Here's how the part is built. I have some questions about the finished solid (model axes, mm). A direction names the side the tool comes from. Round coordinates to 2 decimals unless told otherwise and drop trailing zeros. Write each loop counter-clockwise with the first axis right and the second up, starting at its lowest first coordinate (ties: lowest second). Pieces come first, ordered by that corner, then holes. Notation, with made-up numbers: M 56,36.5 L 96,36.5 A37 cw 96,73.5 Z; hole C 66.5,83.25 d11. An arc over 180 degrees is marked long. Write item = value, one per line. Start each with the question number.
(1) I want a section at C-C (z = -2). Give the number of separate pieces and of enclosed holes in the cut face, and give its area (3 significant figures).
(2) If we mould it in two halves opening along Y, with no side actions, what happens to faces 4 (the flat face through (0, 7, 2)), 5 (the flat face through (-13, 1.55, 1)), 6 (the flat face through (-12.1, 5, -2)), 7 (the flat face through (0, 10, -2))? For each: released by +Y, released by -Y, zero draft, split by the parting line, or undercut.
(3) I want a section at A-A (x = 7). List the corners of the cut face in (y, z) for me.
(4) I want a section at D-D (x = 16). List the corners of the cut face in (y, z) for me, and give its area (3 significant figures).
(5) I want a section at B-B (y = -4.75). List the corners of the cut face in (x, z) for me, and give its area (3 significant figures).
(6) I need wall thicknesses on line 1 along X through (y, z) = (7.55, -2); line 2 along X through (y, z) = (-8.55, -2); line 3 along X through (y, z) = (5, -4.25). Which ranges of each line are inside material? Lowest first, please.
(7) Will this pin go through, and if not, where does the flat tip stop? pin 1 Ø4.5 at (x, y) = (-14.5, 1) entering from -Z.
(8) On a 3-axis mill with a long thin cutter (end or side, diameter ignored), from which of +Z, -Z, +X, -X, +Y, -Y can I reach the whole of each face in a straight line? I mean faces 1 (the flat face through (0, -6.2, 1)), 2 (the flat face through (0, 8.02, -3)), 3 (the flat face through (0, -10, -2)). Say none if no direction works.
```python
from build123d import *

# Parameters (mm, degrees)
SKETCH_1_W          = 40
SKETCH_1_H          = 20
EXTRUDE_1_DEPTH     = 2
SKETCH_2_W          = 24.2
SKETCH_2_H          = 12.4
CUT_EXTRUDE_1_DEPTH = 2
SKETCH_3_W          = 2
SKETCH_3_H          = 20
EXTRUDE_2_DEPTH     = 6
SKETCH_5_W          = 36
SKETCH_5_H          = 1.98
EXTRUDE_3_DEPTH     = 6
SKETCH_6_W          = 5.9
SKETCH_6_H          = 4
EXTRUDE_4_DEPTH     = 6
SKETCH_7_R          = 1.2
CUT_EXTRUDE_2_DEPTH = 29.91366459


with BuildPart() as part:
    # ｽｹｯﾁ1 → ﾎﾞｽ - 押し出し1 (new body)
    with BuildSketch(Plane.XY):
        Rectangle(SKETCH_1_W, SKETCH_1_H)
    extrude(amount=EXTRUDE_1_DEPTH)

    # ｽｹｯﾁ2 → ｶｯﾄ - 押し出し1 (cut)
    with BuildSketch(Plane.XY.offset(2)):
        Rectangle(SKETCH_2_W, SKETCH_2_H)
        with BuildLine():
            Line((-14, 1.55), (14, 1.55))
            ThreePointArc((14, 1.55), (15.55, 0), (14, -1.55))
            Line((14, -1.55), (-14, -1.55))
            ThreePointArc((-14, -1.55), (-15.55, 0), (-14, 1.55))
        make_face()
    extrude(amount=-CUT_EXTRUDE_1_DEPTH, mode=Mode.SUBTRACT)

    # ｽｹｯﾁ3 → ﾎﾞｽ - 押し出し2 (add)
    with BuildSketch(Plane(origin=(0, 0, 0), x_dir=(-1, 0, 0), z_dir=(0, 0, -1))):
        with Locations((19, 0)):
            Rectangle(SKETCH_3_W, SKETCH_3_H)
        with Locations((-19, 0)):
            Rectangle(SKETCH_3_W, SKETCH_3_H)
    extrude(amount=EXTRUDE_2_DEPTH)

    # ｽｹｯﾁ5 → ﾎﾞｽ - 押し出し3 (add)
    with BuildSketch(Plane(origin=(0, 0, 0), x_dir=(-1, 0, 0), z_dir=(0, 0, -1))):
        with Locations((0, 9.01)):
            Rectangle(SKETCH_5_W, SKETCH_5_H)
        with Locations((0, -9.01)):
            Rectangle(SKETCH_5_W, SKETCH_5_H)
    extrude(amount=EXTRUDE_3_DEPTH)

    # ｽｹｯﾁ6 → ﾎﾞｽ - 押し出し4 (add)
    with BuildSketch(Plane(origin=(0, 0, 0), x_dir=(-1, 0, 0), z_dir=(0, 0, -1))):
        with Locations((-15.05, 6.02)):
            Rectangle(SKETCH_6_W, SKETCH_6_H)
        with Locations((15.05, 6.02)):
            Rectangle(SKETCH_6_W, SKETCH_6_H)
        with Locations((15.05, -6.02)):
            Rectangle(SKETCH_6_W, SKETCH_6_H)
        with Locations((-15.05, -6.02)):
            Rectangle(SKETCH_6_W, SKETCH_6_H)
    extrude(amount=EXTRUDE_4_DEPTH)

    # ｽｹｯﾁ7 → ｶｯﾄ - 押し出し2 (cut, through all)
    with BuildSketch(Plane(origin=(0, 10, 0), x_dir=(1, 0, 0), z_dir=(0, 1, 0))):
        with Locations(Location((-16, 2, 0), (0, 0, 270))):
            Circle(SKETCH_7_R)
        with Locations(Location((16, 2, 0), (0, 0, 270))):
            Circle(SKETCH_7_R)
    extrude(amount=-CUT_EXTRUDE_2_DEPTH, mode=Mode.SUBTRACT)


solid = part.part
```
Returned:
q1.separate_pieces = 4
q1.enclosed_holes = 0
q1.area = 260 mm²
q2.face_4 = zero draft
q2.face_5 = undercut
q2.face_6 = undercut
q2.face_7 = released by +Y
q3.outline = M -10,-6 L -8.02,-6 L -8.02,0 L -6.2,0 L -6.2,2 L -10,2 Z; M 6.2,0 L 8.02,0 L 8.02,-6 L 10,-6 L 10,2 L 6.2,2 Z
q4.outline = M -10,-6 L -4.02,-6 L -4.02,-3.2 L -10,-3.2 Z; M -10,-0.8 L -4.02,-0.8 L -4.02,0 L 4.02,0 L 4.02,-0.8 L 10,-0.8 L 10,2 L -10,2 Z; M 4.02,-6 L 10,-6 L 10,-3.2 L 4.02,-3.2 Z
q4.area = 83.1 mm²
q5.outline = M -20,-6 L -12.1,-6 L -12.1,2 L -20,2 Z; M 12.1,-6 L 20,-6 L 20,2 L 12.1,2 Z; hole C -16,-2 d2.4; hole C 16,-2 d2.4
q5.area = 117 mm²
q6.line_1 = -20 to -17.2, -14.8 to -12.1, 12.1 to 14.8, 17.2 to 20
q6.line_2 = -20 to -17.2, -14.8 to 14.8, 17.2 to 20
q6.line_3 = -20 to -12.1, 12.1 to 20
q7.pin_1 = 0
q8.face_1 = +Z, -Z
q8.face_2 = -Z
q8.face_3 = +Z, -Z, +X, -X, -Y
